CAD build for the part. Positions are in the model's coordinates, mm. Face numbers are marked on the shaded views. A direction names the side the tool comes from. Round coordinates to 2 decimals unless told otherwise and drop trailing zeros. Order: outer loops, then holes, each group sorted by start corner. A loop starts at its lowest first (then second) coordinate and runs counter-clockwise, first axis right, second up. Notation, with made-up numbers: M 8.25,34.25 L 12.25,34.25 A33 cw 12.25,66.25 Z; hole C -40,30 d2. An arc over 180 degrees is marked long. Answer as a JSON object with one key per item and string values. Group by question number.
Autodesk Inventor part; units mm, degrees
ref_plane "YZ Plane" through (0, 0, 0) normal (1, 0, 0) x (0, 1, 0)
ref_plane "XZ Plane" through (0, 0, 0) normal (0, 1, 0) x (-1, 0, 0)
ref_plane "XY Plane" through (0, 0, 0) normal (0, 0, 1) x (1, 0, 0)
sketch "Sketch1" plane through (0, 0, 0) normal (0, 1, 0) x (-1, 0, 0)
  line L0 (0, 0) -> (28, 0)
  line L1 (28, 0) -> (28, -22)
  line L2 (28, -22) -> (0, -22)
  line L3 (0, -22) -> (0, 0)
  dimension "d0" = 28
  dimension "d1" = 22
extrude "Extrusion1" add sketch "Sketch1" along normal blind 3
sketch "Sketch2" plane through (0, 3, 0) normal (0, 1, 0) x (1, 0, 0)
  line L0 (-17, 7) -> (-11, 7)
  line L1 (-11, 7) -> (-11, 15)
  line L2 (-11, 15) -> (-17, 15)
  line L3 (-17, 15) -> (-17, 7)
  line L4 (-17, 7) -> (-11, 15) construction
  line L5 (-11, 7) -> (-17, 15) construction
  point P0 (0, 0)
  point P1 (-14, 11)
  dimension "d4" = 6
  dimension "d5" = 8
sketch "Sketch3" plane through (0, 3, 0) normal (0, 1, 0) x (1, 0, 0)
  line L0 (-28, 22) -> (-28, 0)
  line L1 (-28, 11) -> (-23, 11)
  line L2 (0, 0) -> (0, 22)
  line L3 (0, 11) -> (-5, 11)
  circle A0 centre (-5, 11) radius 2.125
  dimension "d6" = 5
  dimension "d7" = 5
  dimension "d8" = 4.25
extrude "Extrusion2" cut sketch "Sketch3" against normal through all
pattern_linear "Rectangular Pattern1" count 3 spacing 6 along (0, 0, 1) count 2 spacing 18 along (-1, 0, 0) of "Extrusion2" first direction both ways yes
sketch "Sketch5" plane through (0, 3, 0) normal (0, 1, 0) x (1, 0, 0)
  line L0 (0, 22) -> (-28, 22)
  line L1 (-19, 0) -> (-9, 0)
  line L2 (-9, 0) -> (-9, 22)
  line L3 (-9, 22) -> (-19, 22)
  line L4 (-19, 22) -> (-19, 0)
  line L5 (-19, 0) -> (-9, 22) construction
  line L6 (-9, 0) -> (-19, 22) construction
  point P0 (0, 0)
  point P1 (-14, 11)
  dimension "d17" = 10
extrude "Extrusion3" add sketch "Sketch5" along normal blind 15
sketch "Sketch6" plane through (-28, 0, 0) normal (0, 0, 1) x (1, 0, 0)
  line L0 (19, 3) -> (17, 3)
  line L1 (9, 3) -> (9, 18)
  line L2 (9, 3) -> (11, 3)
  line L3 (0, 0) -> (28, 0)
  line L4 (17, 3) -> (11, 3)
  line L5 (11, 3) -> (11, 0)
  line L6 (11, 0) -> (17, 0)
  line L7 (17, 0) -> (17, 3)
  dimension "d20" = 2
  dimension "d21" = 2
extrude "Extrusion4" cut sketch "Sketch6" against normal through all
sketch "Sketch7" plane through (-9, 3, 0) normal (1, 0, 0) x (0, 0, -1)
  line L0 (0, 15) -> (7, 15)
  line L1 (22, 15) -> (0, 15)
  line L2 (22, 15) -> (15, 15)
  line L3 (0, 0) -> (0, 15)
  line L4 (7, 15) -> (0, 15)
  line L5 (0, 15) -> (0, 3)
  line L6 (0, 3) -> (7, 3)
  line L7 (7, 3) -> (7, 15)
  line L8 (22, 15) -> (15, 15)
  line L9 (15, 15) -> (15, 3)
  line L10 (15, 3) -> (22, 3)
  line L11 (22, 3) -> (22, 15)
  point P0 (0, -3)
  dimension "d24" = 7
  dimension "d25" = 7
  dimension "d26" = 12
extrude "Extrusion5" cut sketch "Sketch7" against normal through all
sketch "Sketch8" plane through (-9, 6, -15) normal (0, 0, -1) x (-1, 0, 0)
  line L0 (0, 12) -> (10, 12)
  line L1 (5, 12) -> (5, 6)
  line L2 (10, 12) -> (10, 0)
  line L3 (10, 6) -> (6, 6)
  line L4 (0, 0) -> (0, 12)
  line L5 (0, 6) -> (4, 6)
  line L6 (2, 3) -> (8, 3)
  line L7 (8, 3) -> (8, 9)
  line L8 (8, 9) -> (2, 9)
  line L9 (2, 9) -> (2, 3)
  line L10 (2, 3) -> (8, 9) construction
  line L11 (8, 3) -> (2, 9) construction
  point P0 (-9, -6)
  dimension "d29" = 6
  dimension "d30" = 4
  dimension "d31" = 4
extrude "Extrusion6" cut sketch "Sketch8" against normal through all contours L8 L7 L6 L9
fillet "Fillet1" radius 3 1 edges at (-14, 15, -7)
fillet "Fillet2" radius 3 1 edges at (-14, 15, -15)
sketch "Sketch9" plane through (0, 18, 0) normal (0, 1, 0) x (1, 0, 0)
  line L0 (-9, 7) -> (-19, 7)
  line L1 (-19, 7) -> (-19, 15)
  line L2 (-19, 15) -> (-9, 15)
  line L3 (-9, 15) -> (-9, 7)
  line L4 (-9, 7) -> (-19, 15) construction
  line L5 (-19, 7) -> (-9, 15) construction
  point P0 (0, 0)
  point P1 (-14, 11)
extrude "Extrusion7" add sketch "Sketch9" along normal blind 2
properties part number "ClawAttach"
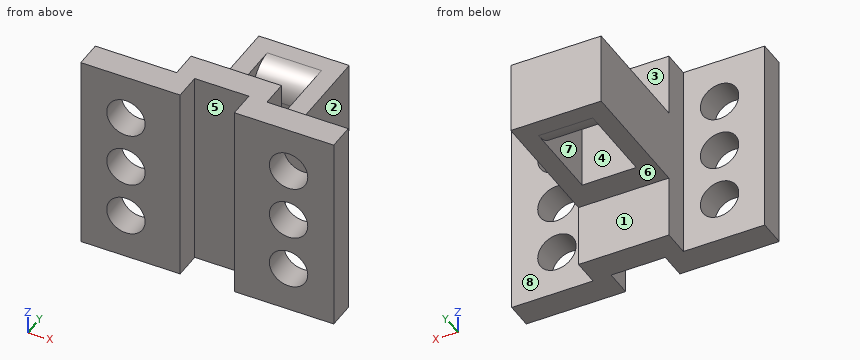
Item 1: Cut at B-B, the plane x = -23. Give the cut face in (y, z) (3 decimals), and give its area (4 significant figures).
Item 2: Drill centre lines: line 1 (Z direction, x = -23, y = 0.8) (3 decimals); line 2 (X direction, y = 0.9, z = -17) (3 decimals); line 3 (Z direction, x = -21.25, y = 2.5). Where is each one in solid material? Low to high. Write a range as [from, to].
Item 3: Flat gauge pins, fed straight in: pin 1 Ø1.8 at (x, z) = (-14, -14) entering from -Y; pin 2 Ø10 at (x, y) = (-10, 14) entering from -Z; pin 3 Ø9 at (y, z) = (12, -11) entering from -X; pin 4 Ø2.5 at (x, z) = (-5, -11) entering from +Y. Where does each tip first touch, or does it go through?
Item 4: Cut at C-C, the plane y = 14.25. Give the cut face in (x, z), and give its area (3 significant figures).
Item 5: 3-axis set-ups, long thin cutter, end or side, ignore diameter. For the marked faces 1, 2, 3, 4 and 5: which of +Z, -Z, +X, -X, +Y, -Y reach the whole face in a straight line?
Item 6: Two-plate mould, pull along Y, no slides. Class the marked faces 6, 7 and 8: +Y half, -Y half, draft (parallel to the pull), parting line (faces both ways), or undercut.
Item 7: Cut at D-D, the plane z = -5. Give the cut face in (x, y) (3 decimals), and give its area (3 significant figures).
Item 8: Cut at A-A, the plane z = -11. Give the cut face in (x, y) (3 decimals), and give its area (4 significant figures).
Response values:
{
 "1": {"outline": "M 0,-22 L 3,-22 L 3,-19.125 L 0,-19.125 Z; M 0,-14.875 L 3,-14.875 L 3,-13.125 L 0,-13.125 Z; M 0,-8.875 L 3,-8.875 L 3,-7.125 L 0,-7.125 Z; M 0,-2.875 L 3,-2.875 L 3,0 L 0,0 Z", "area": "27.75 mm^2"},
 "2": {"line 1": "[-22, -19.125], [-14.875, -13.125], [-8.875, -7.125], [-2.875, 0]", "line 2": "[-28, -25.125], [-20.875, -17], [-11, -7.125], [-2.875, 0]", "line 3": "[-22, -18.21], [-15.79, -12.21], [-9.79, -6.21], [-3.79, 0]"},
 "3": {"pin 1": "y = 3", "pin 2": "z = -15", "pin 3": "x = -19", "pin 4": "through"},
 "4": {"outline": "M -19,-15 L -17,-15 L -17,-7 L -19,-7 Z; M -11,-15 L -9,-15 L -9,-7 L -11,-7 Z", "area": "32.0 mm^2"},
 "5": {"face 1": "-Z, +X, -X, +Y", "face 2": "+Z, -Z, +X, +Y", "face 3": "+Z, +X, -X, +Y", "face 4": "+Z, -Z", "face 5": "+Z, -Z, -Y"},
 "6": {"face 6": "draft", "face 7": "undercut", "face 8": "+Y half"},
 "7": {"outline": "M -28,0 L -25.125,0 L -25.125,3 L -28,3 Z; M -20.875,0 L -17,0 L -17,3 L -11,3 L -11,0 L -7.125,0 L -7.125,3 L -9,3 L -9,6 L -19,6 L -19,3 L -20.875,3 Z; M -2.875,0 L 0,0 L 0,3 L -2.875,3 Z", "area": "70.5 mm^2"},
 "8": {"outline": "M -28,0 L -25.125,0 L -25.125,3 L -28,3 Z; M -20.875,0 L -17,0 L -17,3 L -11,3 L -11,0 L -7.125,0 L -7.125,3 L -9,3 L -9,20 L -19,20 L -19,3 L -20.875,3 Z; M -2.875,0 L 0,0 L 0,3 L -2.875,3 Z; hole M -17,9 L -11,9 L -11,15 L -17,15 Z", "area": "174.5 mm^2"}
}
